Work out the finished part from the listing and answer in its coordinate system (mm). Round coordinates to 2 decimals unless told otherwise and drop trailing zeros. Loops run counter-clockwise (first coordinate to the right, second up) from the corner with the lowest first, then second, coordinate; pieces in that order, holes last. Notation, with made-up numbers: (21, 2) -> (25, 2) arc R16 ccw to (25, 19) -> close; hole circle Ø9 at (-36, 50.5). An arc over 180 degrees is marked (long way). Use one line per item in the form item = value.
```python
from build123d import *

# Parameters (mm, degrees)
SKETCH1_R           = 0.375
BOSS_EXTRUDE1_DEPTH = 0.1


with BuildPart() as part:
    # Sketch1 → Boss-Extrude1 (new body, symmetric)
    with BuildSketch(Plane.XY):
        with BuildLine():
            Line((-4, 8.75), (-0.829156198, 8.75))
            ThreePointArc((-0.829156198, 8.75), (0, 11.5), (0.829156198, 8.75))
            Line((0.829156198, 8.75), (4, 8.75))
            Line((4, 8.75), (4, 8.25))
            Line((4, 8.25), (-0.6875, -7.5))
            Line((-0.6875, -7.5), (-0.6875, -8.666829437))
            ThreePointArc((-0.6875, -8.666829437), (0.960377242, -11.152248043), (-1.1875, -9.083570106))
            Line((-1.1875, -9.083570106), (-1.1875, -7.427173711))
            Line((-1.1875, -7.427173711), (3.478325509, 8.25))
            Line((3.478325509, 8.25), (-4, 8.25))
            Line((-4, 8.25), (-4, 8.75))
        make_face()
        with Locations((0, 10)):
            Circle(SKETCH1_R, mode=Mode.SUBTRACT)
        with Locations((0, -10)):
            Circle(SKETCH1_R, mode=Mode.SUBTRACT)
    extrude(amount=BOSS_EXTRUDE1_DEPTH, both=True)


solid = part.part
```
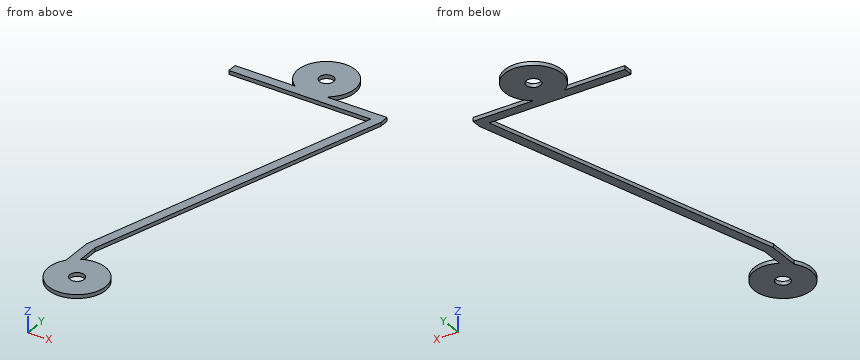
(1) Find section C-C, the plane x = 0. Write down the section's boundary in (y, z) (3 decimals), then the cut area to 3 significant figures.
Completed:
outline = (-11.5, -0.1) -> (-10.375, -0.1) -> (-10.375, 0.1) -> (-11.5, 0.1) -> close; (-9.625, -0.1) -> (-8.5, -0.1) -> (-8.5, 0.1) -> (-9.625, 0.1) -> close; (-5.19, -0.1) -> (-3.437, -0.1) -> (-3.437, 0.1) -> (-5.19, 0.1) -> close; (8.25, -0.1) -> (9.625, -0.1) -> (9.625, 0.1) -> (8.25, 0.1) -> close; (10.375, -0.1) -> (11.5, -0.1) -> (11.5, 0.1) -> (10.375, 0.1) -> close
area = 1.30 mm2
(2) Consider L1, parallel to Y at x = -2.5, z = 0.05; L2, parallel to X at y = -7.75, z = -0.05; L3, parallel to X at y = -6, z = 0.05. Determine where each line is inside the solid, lowest interval first.
Completed:
L1 = 8.25 to 8.75
L2 = -1.19 to -0.69
L3 = -0.76 to -0.24
(3) Find section A-A, the plane y = 10. Write down the section's boundary in (x, z) (3 decimals), then the cut area to 3 significant figures.
Completed:
outline = (-1.5, -0.1) -> (-0.375, -0.1) -> (-0.375, 0.1) -> (-1.5, 0.1) -> close; (0.375, -0.1) -> (1.5, -0.1) -> (1.5, 0.1) -> (0.375, 0.1) -> close
area = 0.450 mm2
(4) Find section B-B, the plane z = -0.05. State how many separate pieces and enclosed holes the cut face has, then the cut area to 3 significant figures.
Completed:
separate_pieces = 1
enclosed_holes = 2
area = 25.9 mm2
(5) Find section D-D, the plane y = -8. Write down the section's boundary in (x, z), then the cut area to 3 significant figures.
Completed:
outline = (-1.19, -0.1) -> (-0.69, -0.1) -> (-0.69, 0.1) -> (-1.19, 0.1) -> close
area = 0.100 mm2
